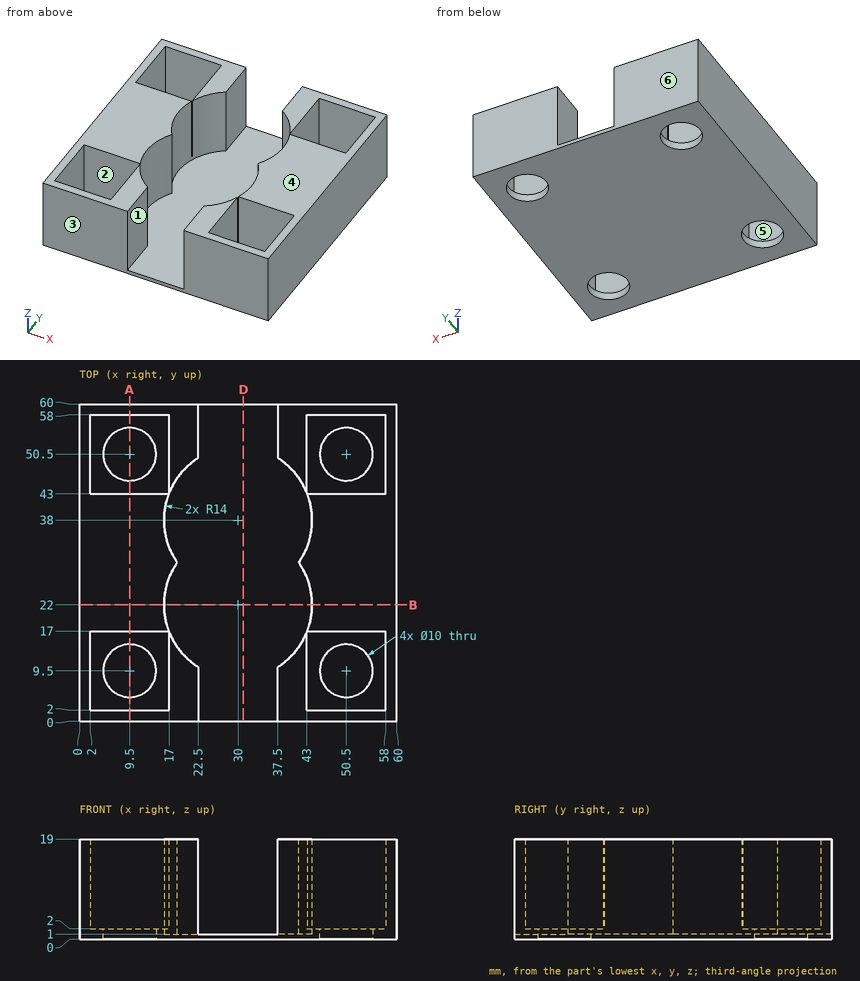
Can you work these out from the drawing? Everything is in mm from the part's minimum corner. A direction names the side the tool comes from. Round coordinates to 2 decimals unless told otherwise and drop trailing zeros. Write each loop counter-clockwise with the first axis right and the second up, starting at its lowest first coordinate (ties: lowest second). Pieces come first, ordered by that corner, then holes.
1. Will this pin go through, and if not, where does the flat tip stop? pin 1 Ø7.5 at (x, y) = (11.5, 50.5) entering from +Z.
2. If we mould it in two halves opening along Y, with no side actions, what happens to the marked faces 4, 5 and 6? For each: released by +Y, released by -Y, zero draft, split by the parting line, or undercut.
3. I need wall thicknesses on L1, parallel to Y at x = 9.5, z = 0.75; L2, parallel to X at y = 55, z = 6.75; L3, parallel to Y at x = 14, z = 11.25. Which ranges of each line are inside material? Lowest first, please.
4. Suppose I cut it at D-D (x = 31). List the corners of the cut face in (y, z) for me.
5. Suppose I cut it at B-B (y = 22). List the corners of the cut face in (x, z) for me, and give its area (3 significant figures).
6. For the marked faces 1, 2 and 3, which set-ups out of +Z, -Z, +X, -X, +Y, -Y let a thin tool reach every point of the face, with its end or its side?
7. Suppose I cut it at A-A (x = 9.5). List the corners of the cut face in (y, z) for me.
Answer sheet:
1. pin 1: stops at z = 2
2. face 4: zero draft
2. face 5: undercut
2. face 6: released by +Y
3. L1: y = 0 to 4.5, 14.5 to 45.5, 55.5 to 60
3. L2: x = 0 to 2, 17 to 22.5, 37.5 to 43, 58 to 60
3. L3: y = 0 to 2, 17 to 43, 58 to 60
4. outline: (0, 0) - (60, 0) - (60, 1) - (0, 1) - close
5. outline: (0, 0) - (60, 0) - (60, 19) - (44, 19) - (44, 1) - (16, 1) - (16, 19) - (0, 19) - close
5. area: 636 mm2
6. face 1: +Z, +Y, -Y
6. face 2: +Z
6. face 3: +Z, -Z, +X, -X, -Y
7. outline: (0, 0) - (4.5, 0) - (4.5, 2) - (2, 2) - (2, 19) - (0, 19) - close; (14.5, 0) - (45.5, 0) - (45.5, 2) - (43, 2) - (43, 19) - (17, 19) - (17, 2) - (14.5, 2) - close; (55.5, 0) - (60, 0) - (60, 19) - (58, 19) - (58, 2) - (55.5, 2) - close
